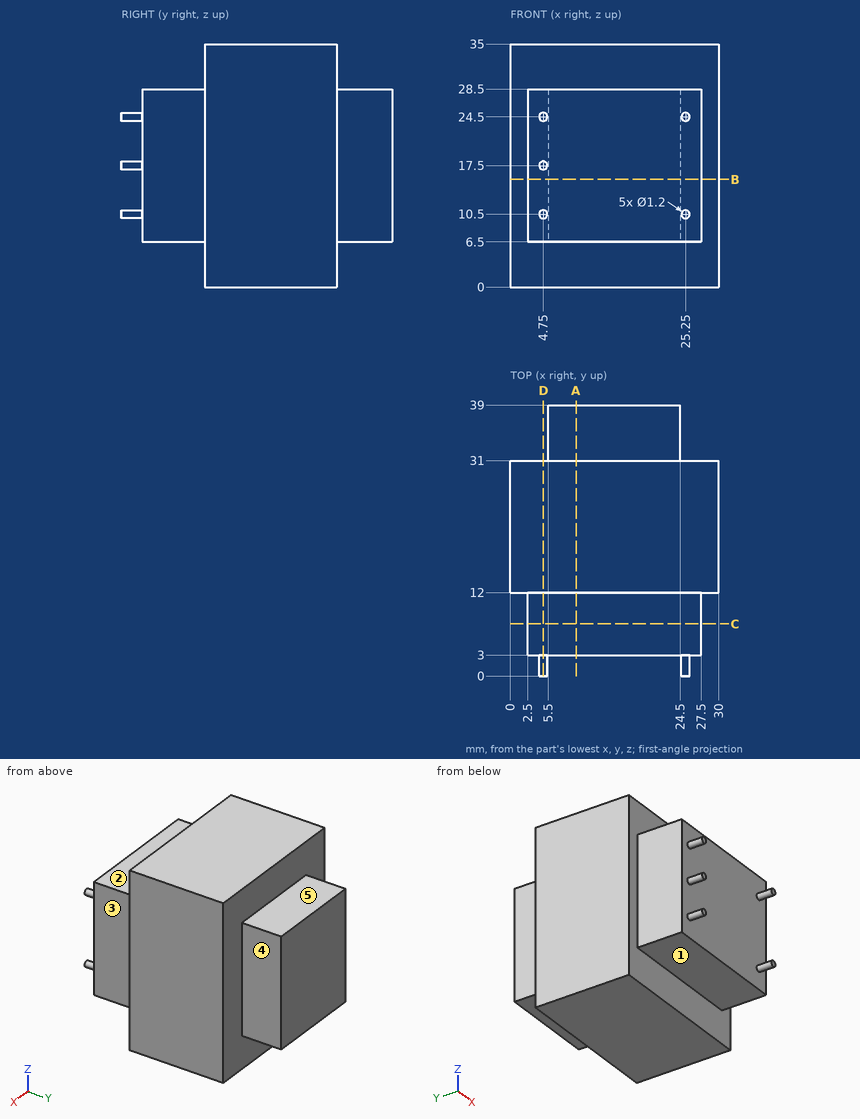
The drawing under review shows one solid part. Ordinate dimensions are in mm from its lowest x, y, z. A direction names the side the tool comes from. Give positions to 0.01 mm unless a question says otherwise; leave off trailing zeros. Order: outer loops, then holes, each group sorted by start corner. A loop starts at its lowest first (then second) coordinate and runs counter-clockwise, first axis right, second up. Notation, with made-up numbers: M 55.25,-19.75 L 74.25,-19.75 A17 ccw 74.25,-2.75 Z; hole C 81.25,-27.5 d6. An arc over 180 degrees is marked long. One line per question, with ' | ' between items. Start each with the question number.
Q1. We need section A-A (x = 9.5). Write out the cut boundary in (y, z).
Q2. Machinability: for the marked faces 1, 2, 3, 4 and 5, which of the approach directions +Z, -Z, +X, -X, +Y, -Y give a long, thin tool a straight path to every point of the face, cutting with its end or side? Answer none if there is none.
Q3. We need section B-B (z = 15.5). Write out the cut boundary in (x, y), plus the area to 3 significant figures.
Q4. For pin 1 Ø10 at (y, z) = (8, 29.5) entering from +X; pin 2 Ø4.5 at (x, y) = (13, 9) entering from -Z; pin 3 Ø3 at (y, z) = (7, 10.5) entering from -X; pin 4 Ø2 at (x, y) = (16.5, 9) entering from +Z, all flat-tipped, find the tip position at first contact; note any pin that passes through.
Q5. We need section C-C (y = 7.5). Write out the cut boundary in (x, z).
Q6. We need section D-D (x = 4.75). Write out the cut boundary in (y, z).
Q7. For L1, parallel to Y at x = 10.25, z = 8; L2, parallel to Y at x = 25.5, z = 9.5; L3, parallel to Z at x = 6.5, y = 4, list the stretches that pass through material, from the lowest coordinate up. Write a range as [from, to].
Returned:
1) outline: M 3,6.5 L 12,6.5 L 12,0 L 31,0 L 31,6.5 L 39,6.5 L 39,28.5 L 31,28.5 L 31,35 L 12,35 L 12,28.5 L 3,28.5 Z
2) face 1: -Z, +X, -X, -Y | face 2: +Z, +X, -X, -Y | face 3: +Z, -Z, +X, -Y | face 4: +Z, -Z, +X, +Y | face 5: +Z, +X, -X, +Y
3) outline: M 0,12 L 2.5,12 L 2.5,3 L 27.5,3 L 27.5,12 L 30,12 L 30,31 L 24.5,31 L 24.5,39 L 5.5,39 L 5.5,31 L 0,31 Z | area: 947 mm2
4) pin 1: x = 30 | pin 2: z = 6.5 | pin 3: x = 2.5 | pin 4: z = 28.5
5) outline: M 2.5,6.5 L 27.5,6.5 L 27.5,28.5 L 2.5,28.5 Z
6) outline: M 0,9.9 L 3,9.9 L 3,6.5 L 12,6.5 L 12,0 L 31,0 L 31,35 L 12,35 L 12,28.5 L 3,28.5 L 3,25.1 L 0,25.1 L 0,23.9 L 3,23.9 L 3,18.1 L 0,18.1 L 0,16.9 L 3,16.9 L 3,11.1 L 0,11.1 Z
7) L1: [3, 39] | L2: [3, 31] | L3: [6.5, 28.5]
